The listing builds one solid part. Answer for the finished solid, in the listing's coordinates (mm). A direction names the side the tool comes from. Round coordinates to 2 decimals unless told otherwise and drop trailing zeros. Write each loop counter-clockwise with the first axis right and the second up, starting at its lowest first coordinate (ties: lowest second). Pieces come first, ordered by that corner, then holes. Notation, with made-up numbers: (-29, 30.25) - (20, 30.25) arc R26 ccw to (20, 66.25) - close; hole circle Ø2 at (37, -12.75). An arc over 180 degrees is marked (long way). Answer in a Markdown table with one row per item.
from build123d import *

# Parameters (mm, degrees)
SKETCH1_W           = 12
SKETCH1_H           = 15
BOSS_EXTRUDE1_DEPTH = 9
SKETCH2_W           = 3.25
SKETCH2_H           = 4.8
BOSS_EXTRUDE2_DEPTH = 3
SKETCH3_R           = 3
CUT_EXTRUDE1_DEPTH  = 501.290165804
FILLET1_R           = 2
SKETCH4_R           = 1
CUT_EXTRUDE2_DEPTH  = 15


with BuildPart() as part:
    # Sketch1 → Boss-Extrude1 (new body)
    with BuildSketch(Plane.XY.offset(20)):
        with Locations((231, 433)):
            Rectangle(SKETCH1_W, SKETCH1_H)
    extrude(amount=BOSS_EXTRUDE1_DEPTH)

    # Sketch2 → Boss-Extrude2 (add)
    with BuildSketch(Plane.XY.offset(29)):
        with Locations((235.325, 438.1)):
            Rectangle(SKETCH2_W, SKETCH2_H)
        with Locations((226.625, 438.1)):
            Rectangle(SKETCH2_W, SKETCH2_H)
        with Locations((235.325, 427.9)):
            Rectangle(SKETCH2_W, SKETCH2_H)
        with Locations((226.625, 427.9)):
            Rectangle(SKETCH2_W, SKETCH2_H)
    extrude(amount=BOSS_EXTRUDE2_DEPTH)

    # Sketch3 → Cut-Extrude1 (cut, through all)
    with BuildSketch(Plane.XY.offset(29)):
        with Locations((231.026544884, 432.975080758)):
            Circle(SKETCH3_R)
    extrude(amount=-CUT_EXTRUDE1_DEPTH, mode=Mode.SUBTRACT)

    # Fillet1
    fillet1_edges = [part.edges().sort_by_distance(p)[0] for p in [
        (228.25, 435.7, 30.5),
        (233.7, 435.7, 30.5),
        (233.7, 430.3, 30.5),
        (228.25, 430.3, 30.5),
    ]]
    fillet(fillet1_edges, radius=FILLET1_R)

    # Sketch4 → Cut-Extrude2 (cut)
    with BuildSketch(Plane(origin=(0, 425.5, 0), x_dir=(-1, 0, 0), z_dir=(0, -1, 0))):
        with Locations(Location((-227.379453892, -23, 0), (0, 0, 90))):
            Circle(SKETCH4_R)
        with Locations(Location((-234.179453892, -23, 0), (0, 0, 90))):
            Circle(SKETCH4_R)
    extrude(amount=-CUT_EXTRUDE2_DEPTH, mode=Mode.SUBTRACT)


solid = part.part
(1) Find the intervals of material crossed by line 1 (X direction, y = 429.75, z = 23); line 2 (Y direction, x = 226, z = 30.25); line 3 (Z direction, x = 234, y = 438.75), in increasing order.
Checked values:
| item | result |
|---|---|
| line 1 | x = 225 to 226.38, 228.38 to 233.18, 235.18 to 237 |
| line 2 | y = 425.5 to 430.3, 435.7 to 440.5 |
| line 3 | z = 20 to 22.02, 23.98 to 32 |
(2) Section D-D (z = 22.75) is taken. Give the vertices of the cut face in (x, y), and give its area (3 significant figures).
Checked values:
| item | result |
|---|---|
| outline | (225, 425.5) - (226.41, 425.5) - (226.41, 440.5) - (225, 440.5) - close; (228.35, 425.5) - (233.21, 425.5) - (233.21, 430.92) arc R3 cw to (228.35, 431.62) - close; (228.35, 434.33) arc R3 cw to (233.21, 435.03) - (233.21, 440.5) - (228.35, 440.5) - close; (235.15, 425.5) - (237, 425.5) - (237, 440.5) - (235.15, 440.5) - close |
| area | 96.5 mm2 |
(3) Section A-A (z = 31) is taken. Give the vertices of the cut face in (x, y).
Checked values:
| item | result |
|---|---|
| outline | (225, 425.5) - (228.25, 425.5) - (228.25, 428.3) arc R2 ccw to (226.25, 430.3) - (225, 430.3) - close; (225, 435.7) - (226.25, 435.7) arc R2 ccw to (228.25, 437.7) - (228.25, 440.5) - (225, 440.5) - close; (233.7, 425.5) - (236.95, 425.5) - (236.95, 430.3) - (235.7, 430.3) arc R2 ccw to (233.7, 428.3) - close; (233.7, 437.7) arc R2 ccw to (235.7, 435.7) - (236.95, 435.7) - (236.95, 440.5) - (233.7, 440.5) - close |
(4) Flat-ended cylindrical pins translate along their axes: pin 1 (2.5 mm diameter, centred on y = 428, z = 30.5, fed in from +X); pin 2 (3 mm diameter, centred on x = 228, y = 432.5, fed in from +Z). Find the tip coordinate at first contact, or state that the pin passes through.
Checked values:
| item | result |
|---|---|
| pin 1 | stops at x = 236.95 |
| pin 2 | stops at z = 29 |
(5) Section B-B (y = 430.5) is taken. Give the vertices of the cut face in (x, z).
Checked values:
| item | result |
|---|---|
| outline | (225, 20) - (229.33, 20) - (229.33, 29) - (225, 29) - close; (232.72, 20) - (237, 20) - (237, 29) - (232.72, 29) - close; hole circle Ø2 at (227.38, 23); hole circle Ø2 at (234.18, 23) |
(6) Section C-C (x = 227) is taken. Give the vertices of the cut face in (y, z), and give its area (3 significant figures).
Checked values:
| item | result |
|---|---|
| outline | (425.5, 20) - (440.5, 20) - (440.5, 22.07) - (425.5, 22.07) - close; (425.5, 23.93) - (440.5, 23.93) - (440.5, 32) - (435.85, 32) - (435.85, 29) - (430.15, 29) - (430.15, 32) - (425.5, 32) - close |
| area | 135 mm2 |
(7) For faces 1 (the cylindrical face through (234.27, 436.3, 30.52)), 2 (the flat face through (233.7, 439, 30)), 3 (the flat face through (226, 430.3, 30)), 4 (the flat face through (227, 428, 32)), determine the directions among +Z, -Z, +X, -X, +Y, -Y from which every point of the face is accessible in a straight line to the end or side of a thin tool.
Checked values:
| item | result |
|---|---|
| face 1 | +Z |
| face 2 | +Z, +Y, -Y |
| face 3 | +Z, +X, -X |
| face 4 | +Z, +X, -X, +Y, -Y |
(8) For a pull along X with two mould halves and no side action, classify faces 5 (the flat face through (236.95, 428, 30)), 6 (the flat face through (228.25, 439, 30)), 7 (the flat face through (226, 435.7, 30)) as pulls with the +X half, pulls with the -X half, needs draft (parallel to the pull), parting line crosses it, or undercut.
Checked values:
| item | result |
|---|---|
| face 5 | pulls with the +X half |
| face 6 | undercut |
| face 7 | needs draft |
